Verification items for the finished model (mm, model axes). Coordinates: 2 decimals unless noted, no trailing zeros. Order: outer loops, then holes, each group sorted by start corner. A loop starts at its lowest first (then second) coordinate and runs counter-clockwise, first axis right, second up. Notation, with made-up numbers: (23.25, -33.75) -> (40.25, -33.75) arc R9 cw to (40.25, -16.75) -> close; hole circle Ø5 at (14, 68). An arc over 180 degrees is marked (long way). Answer as CSV lines item,"result".
```python
from build123d import *

# Parameters (mm, degrees)
BOSS_EXTRUDE1_DEPTH                            = 125
SKETCH3_R                                      = 2
CUT_EXTRUDE2_DEPTH                             = 100
LPATTERN1_COUNT                                = 28
LPATTERN1_PITCH                                = 8
FILLET1_R                                      = 1
CSK_FOR_M4_FLAT_HEAD_MACHINE_SCREW1_AT_2_COUNT = 2
CSK_FOR_M4_FLAT_HEAD_MACHINE_SCREW1_AT_2_PITCH = 75


with BuildPart() as part:
    # Sketch1 → Boss-Extrude1 (new body)
    with BuildSketch(Plane.XY):
        Polygon((-9, 0), (9, 0), (11.309401077, 4), (9, 8), (12.5, 8), (12.5, -3), (-12.5, -3), (-12.5, 8), (-9, 8), (-11.309401077, 4), align=None)
    extrude(amount=-BOSS_EXTRUDE1_DEPTH)

    # Sketch3 → Cut-Extrude2 (cut)
    with BuildSketch(Plane(origin=(12.5, 0, 0), x_dir=(0, 0, -1), z_dir=(1, 0, 0))):
        with Locations((8, 4)):
            Circle(SKETCH3_R)
    cut_extrude2 = extrude(amount=-CUT_EXTRUDE2_DEPTH, mode=Mode.SUBTRACT)

    # LPattern1: Cut-Extrude2 ×28
    with Locations(*[(0, 0, -i * LPATTERN1_PITCH) for i in range(1, LPATTERN1_COUNT)]):
        add(cut_extrude2, mode=Mode.SUBTRACT)

    # Fillet1
    fillet1_edges = [part.edges().sort_by_distance(p)[0] for p in [
        (12.5, -3, -62.5),
        (-12.5, -3, -62.5),
    ]]
    fillet(fillet1_edges, radius=FILLET1_R)

    # Sketch4 → CSK for M4 Flat Head Machine Screw1 (revolve, cut)
    with BuildSketch(Plane(origin=(0, 0, -100), x_dir=(0, 0, 1), z_dir=(1, 0, 0))):
        Polygon((0, 0), (0, 3), (2.25, 3), (2.25, 2.45), (4.7, 0), align=None)
    csk_for_m4_flat_head_machine_screw1 = revolve(axis=Axis((0, 6.35, -100), (0, -1, 0)), mode=Mode.SUBTRACT)

    # CSK for M4 Flat Head Machine Screw1 at 2: CSK for M4 Flat Head Machine Screw1 ×2
    with Locations(*[(0, 0, i * CSK_FOR_M4_FLAT_HEAD_MACHINE_SCREW1_AT_2_PITCH) for i in range(1, CSK_FOR_M4_FLAT_HEAD_MACHINE_SCREW1_AT_2_COUNT)]):
        add(csk_for_m4_flat_head_machine_screw1, mode=Mode.SUBTRACT)


solid = part.part
```
Item 1: Depth check by flat-ended pin: pin 1 Ø1 at (x, z) = (0, -49) entering from +Y. Enter the tip coordinate at first touch or a pass-through.
Answer list:
pin 1,"y = 0"
Item 2: Section check B-B, the plane x = 0. Record the boundary of the cut face in (y, z).
Answer list:
outline,"(-3, -125) -> (0, -125) -> (0, -104.7) -> (-2.45, -102.25) -> (-3, -102.25) -> close; (-3, -97.75) -> (-2.45, -97.75) -> (0, -95.3) -> (0, -29.7) -> (-2.45, -27.25) -> (-3, -27.25) -> close; (-3, -22.75) -> (-2.45, -22.75) -> (0, -20.3) -> (0, 0) -> (-3, 0) -> close"
Item 3: Section check A-A, the plane z = -8. Record the boundary of the cut face in (x, y).
Answer list:
outline,"(-12.5, -2) arc R1 ccw to (-11.5, -3) -> (11.5, -3) arc R1 ccw to (12.5, -2) -> (12.5, 2) -> (10.15, 2) -> (9, 0) -> (-9, 0) -> (-10.15, 2) -> (-12.5, 2) -> close; (-12.5, 6) -> (-10.15, 6) -> (-9, 8) -> (-12.5, 8) -> close; (9, 8) -> (10.15, 6) -> (12.5, 6) -> (12.5, 8) -> close"
Item 4: Section check C-C, the plane z = -100. Record the boundary of the cut face in (x, y).
Answer list:
outline,"(-12.5, -2) arc R1 ccw to (-11.5, -3) -> (-2.25, -3) -> (-2.25, -2.45) -> (-4.7, 0) -> (-9, 0) -> (-11.31, 4) -> (-9, 8) -> (-12.5, 8) -> close; (2.25, -3) -> (11.5, -3) arc R1 ccw to (12.5, -2) -> (12.5, 8) -> (9, 8) -> (11.31, 4) -> (9, 0) -> (4.7, 0) -> (2.25, -2.45) -> close"
Item 5: Release check for a two-part mould opening along Z. For faces 1 (the cylindrical face through (12, 6, -48)), 2 (the flat face through (0, -1, -125)), 3 (the flat face through (-9.882, 6.472, -61.625)) record: +Z half, -Z half, draft (parallel to the pull), parting line (faces both ways), or undercut.
Answer list:
face 1,"undercut"
face 2,"-Z half"
face 3,"draft"
Item 6: Section check D-D, the plane x = -6. Record the boundary of the cut face in (y, z).
Answer list:
outline,"(-3, -125) -> (0, -125) -> (0, 0) -> (-3, 0) -> close"
Item 7: Thickness scan on line 1 (Z direction, x = 1.5, y = -2.25); line 2 (Y direction, x = -5.75, z = -43); line 3 (Y direction, x = 11.25, z = -58.5). Record the ranges inside material, lowest first.
Answer list:
line 1,"-125 to -101.94, -98.06 to -26.94, -23.06 to 0"
line 2,"-3 to 0"
line 3,"-3 to 3.9, 4.1 to 8"
